The model under review builds one solid part; all positions refer to its coordinate system, in mm. A direction names the side the tool comes from. Coordinates: 2 decimals unless noted, no trailing zeros. Write each loop counter-clockwise with the first axis right and the second up, starting at its lowest first coordinate (ties: lowest second). Pieces come first, ordered by that corner, then holes.
1) Machinability: for faces 4 (the flat face through (14, 5, 6)), 5 (the flat face through (0, 169.27, 0)), which of the approach directions +Z, -Z, +X, -X, +Y, -Y give a long, thin tool a straight path to every point of the face, cutting with its end or side? Answer none if there is none.
2) For P1, Ø12, axis at x = 15, y = 143, coming from the +Z side; P2, Ø5, axis at x = -19, y = 40, coming from the -Z side; P3, Ø8.5, axis at x = 22.5, z = 0, coming from the +Y side; P4, Ø17, axis at y = 154.27, z = 0, coming from the +X side, all flat-tipped, find the tip position at first contact; note any pin that passes through.
3) Add section C-C, the plane x = 7.5. State the section outline as (y, z) points, then the cut area to 3 significant figures.
4) Mouldability with a two-part tool opening along Z and no side actions: class faces 1 (the cylindrical face through (18.84, 2.54, -0.81)), 2 (the cylindrical face through (1.32, 2.46, -29.97)), 3 (the flat face through (0, 0, 0)) as released by +Z, released by -Z, zero draft, split by the parting line, or undercut.
5) Add section D-D, the plane y = 115.5. State the section outline as (x, z) points.
6) Add section A-A, the plane z = 20.5. State the section outline as (x, y) points, then the cut area to 3 significant figures.
7) For line 1 (X direction, y = 2.05, z = 0); line 2 (Y direction, x = 3.5, z = 0); line 3 (Y direction, x = 17.5, z = 20.5), list the stretches that pass through material, from the lowest coordinate up.
8) Add section B-B, the plane x = -22.5. State the section outline as (y, z) points, then the cut area to 3 significant figures.
from build123d import *

# Parameters (mm, degrees)
SKETCH1_R           = 30
BOSS_EXTRUDE1_DEPTH = 5
SKETCH2_R           = 3.75
CUT_EXTRUDE1_DEPTH  = 5
SKETCH3_R           = 15
BOSS_EXTRUDE2_DEPTH = 164.27
SKETCH4_R           = 7.5
CUT_EXTRUDE2_DEPTH  = 178.700120709


with BuildPart() as part:
    # Sketch1 → Boss-Extrude1 (new body)
    with BuildSketch(Plane(origin=(0, 0, 0), x_dir=(1, 0, 0), z_dir=(0, 1, 0))):
        with Locations(Location((0, 0, 0), (0, 0, 270))):
            Circle(SKETCH1_R)
    extrude(amount=BOSS_EXTRUDE1_DEPTH)

    # Sketch2 → Cut-Extrude1 (cut)
    with BuildSketch(Plane(origin=(0, 5, 0), x_dir=(1, 0, 0), z_dir=(0, 1, 0))):
        with Locations(Location((0, 22.5, 0), (0, 0, 270))):
            Circle(SKETCH2_R)
        with Locations(Location((22.5, 0, 0), (0, 0, 270))):
            Circle(SKETCH2_R)
        with Locations(Location((0, -22.5, 0), (0, 0, 270))):
            Circle(SKETCH2_R)
        with Locations(Location((-22.5, 0, 0), (0, 0, 270))):
            Circle(SKETCH2_R)
    extrude(amount=-CUT_EXTRUDE1_DEPTH, mode=Mode.SUBTRACT)

    # Sketch3 → Boss-Extrude2 (add)
    with BuildSketch(Plane(origin=(0, 5, 0), x_dir=(1, 0, 0), z_dir=(0, 1, 0))):
        with Locations(Location((0, 0, 0), (0, 0, 270))):
            Circle(SKETCH3_R)
    extrude(amount=BOSS_EXTRUDE2_DEPTH)

    # Sketch4 → Cut-Extrude2 (cut, through all)
    with BuildSketch(Plane(origin=(15, 0, 0), x_dir=(0, 0, -1), z_dir=(1, 0, 0))):
        with Locations((0, 154.27)):
            Circle(SKETCH4_R)
    extrude(amount=-CUT_EXTRUDE2_DEPTH, mode=Mode.SUBTRACT)


solid = part.part
Geometry results:
1. face 4: +Y
1. face 5: +Z, -Z, +X, -X, +Y
2. P1: stops at z = 12
2. P2: passes through
2. P3: stops at y = 5
2. P4: stops at x = 15
3. outline: (0, -29.05) - (5, -29.05) - (5, -12.99) - (169.27, -12.99) - (169.27, 12.99) - (5, 12.99) - (5, 29.05) - (0, 29.05) - close; hole circle Ø15 at (154.27, 0)
3. area: 4,380 mm2
4. face 1: undercut
4. face 2: split by the parting line
4. face 3: zero draft
5. outline: circle Ø30 at (0, 0)
6. outline: (-21.9, 0) - (-3.17, 0) - (-3.17, 5) - (-21.9, 5) - close; (3.17, 0) - (21.9, 0) - (21.9, 5) - (3.17, 5) - close
6. area: 187 mm2
7. line 1: x = -30 to -26.25, -18.75 to 18.75, 26.25 to 30
7. line 2: y = 0 to 146.77, 161.77 to 169.27
7. line 3: y = 0 to 5
8. outline: (0, -19.84) - (5, -19.84) - (5, -3.75) - (0, -3.75) - close; (0, 3.75) - (5, 3.75) - (5, 19.84) - (0, 19.84) - close
8. area: 161 mm2
